Source: CAD feature listing. Evaluate the final solid. Frame: model axes, mm. A direction names the side the tool comes from. Give positions to 0.01 mm unless a question says otherwise; leave off trailing zeros. Write each loop counter-clockwise with the first axis right and the second up, starting at its lowest first coordinate (ties: lowest second). Pieces come first, ordered by that corner, then holes. Notation, with made-up numbers: (-5.5, 26.25) - (18.5, 26.25) arc R25 ccw to (18.5, 41.25) - close; hole circle Ø6 at (-35.5, 7). An arc over 180 degrees is marked (long way). Answer as a JSON object with one key per item and string values. Group by question number.
from build123d import *

# Parameters (mm, degrees)
SKETCH1_R           = 9.525
BOSS_EXTRUDE1_DEPTH = 63.5
CUT_EXTRUDE2_START  = -56.515
SKETCH3_R           = 9.525
CUT_EXTRUDE2_DEPTH  = 56.515


with BuildPart() as part:
    # Sketch1 → Boss-Extrude1 (new body)
    with BuildSketch(Plane(origin=(0, 0, 0), x_dir=(1, 0, 0), z_dir=(0, 1, 0))):
        with Locations(Location((0, 0, 0), (0, 0, 270))):
            Circle(SKETCH1_R)
        Polygon((7.478995387, 0), (3.739497694, 6.477), (-3.739497694, 6.477), (-7.478995387, 0), (-3.739497694, -6.477), (3.739497694, -6.477), align=None, mode=Mode.SUBTRACT)
    extrude(amount=BOSS_EXTRUDE1_DEPTH)

    # Sketch3 → Cut-Extrude2 (cut)
    with BuildSketch(Plane(origin=(0, 63.5, 0), x_dir=(1, 0, 0), z_dir=(0, 1, 0)).offset(CUT_EXTRUDE2_START)):
        with Locations(Location((0, 0, 0), (0, 0, 270))):
            Circle(SKETCH3_R)
    extrude(amount=CUT_EXTRUDE2_DEPTH, mode=Mode.SUBTRACT)


solid = part.part
Q1. Section D-D on z = 7.5. Return the cut outline in (x, y) (3 decimals), then the cut area to 3 significant figures.
Q2. Section A-A on x = 0. Return the cut outline in (y, z) (3 decimals), then the cut area to 3 significant figures.
Q3. Ray query, probe 1 along Z at (x, y) = (0.25, 1); probe 2 along Z at (x, y) = (-5.75, 2.5); probe 3 along X at (y, z) = (6.75, -6.25). Return the intervals inside material, ascending. Write a range as [from, to].
Q4. Section C-C on z = -3. Return the cut outline in (x, y) (3 decimals).
Q5. Draft query along Z for faces 1 (the cylindrical face through (-5.796, 3.444, -7.559)), 2 (the flat face through (6.5, 6.985, -2.3)), 3 (the flat face through (5.635, 3.444, -3.193)). Return one class per face: released by +Z, released by -Z, zero draft, split by the parting line, or undercut.
Q6. First-contact query: pin 1 Ø1 at (x, y) = (-3, 5.5) entering from +Z. Flat tip, straight axial feed; report the tip coordinate or a pass-through.
Q7. Reachability of faces 4 (the flat face through (0, 3, 6.477)), 5 (the flat face through (6.5, 0, -2.3)) from +Z, -Z, +X, -X, +Y, -Y: full face, straight path, thin tool, end or side. Return the list, or none.
Taken from the geometry:
{
 "1": {"outline": "(-5.872, 0) - (5.872, 0) - (5.872, 6.985) - (-5.872, 6.985) - close", "area": "82.0 mm²"},
 "2": {"outline": "(0, -9.525) - (6.985, -9.525) - (6.985, -6.477) - (0, -6.477) - close; (0, 6.477) - (6.985, 6.477) - (6.985, 9.525) - (0, 9.525) - close", "area": "42.6 mm²"},
 "3": {"probe 1": "z = [-9.52, -6.48], [6.48, 9.52]", "probe 2": "z = [-7.59, -2.99], [2.99, 7.59]", "probe 3": "x = [-7.19, -3.87], [3.87, 7.19]"},
 "4": {"outline": "(-9.04, 0) - (-5.747, 0) - (-5.747, 6.985) - (-9.04, 6.985) - close; (5.747, 0) - (9.04, 0) - (9.04, 6.985) - (5.747, 6.985) - close"},
 "5": {"face 1": "split by the parting line", "face 2": "zero draft", "face 3": "undercut"},
 "6": {"pin 1": "stops at z = 9.19"},
 "7": {"face 4": "+Y, -Y", "face 5": "+Z, -Z, +X, -X, -Y"}
}
